from build123d import *

# Parameters (mm, degrees)
F1_DEPTH = 10


with BuildPart() as f1:
    # F0 (on Front) → F1 (new body)
    with BuildSketch(Plane.XZ):
        with BuildLine():
            Line((-30.2, 0), (0, 0))
            Line((0, 0), (0, 1.4))
            Line((0, 1.4), (-15.1, 1.4))
            Line((-15.1, 1.4), (-15.1, 12.9))
            ThreePointArc((-15.1, 12.9), (-15.246447, 13.253553), (-15.6, 13.4))
            ThreePointArc((-15.6, 13.4), (-15.953553, 13.253553), (-16.1, 12.9))
            Line((-16.1, 12.9), (-16.1, 4.4))
            ThreePointArc((-16.1, 4.4), (-16.97868, 2.27868), (-19.1, 1.4))
            Line((-19.1, 1.4), (-28.8, 1.4))
            ThreePointArc((-28.8, 1.4), (-29.789949, 0.989949), (-30.2, 0))
        make_face()
        with BuildLine():
            Line((0, 1.4), (0, 0))
            Line((0, 0), (30.2, 0))
            ThreePointArc((30.2, 0), (29.789949, 0.989949), (28.8, 1.4))
            Line((28.8, 1.4), (19.1, 1.4))
            ThreePointArc((19.1, 1.4), (16.97868, 2.27868), (16.1, 4.4))
            Line((16.1, 4.4), (16.1, 12.9))
            ThreePointArc((16.1, 12.9), (15.953553, 13.253553), (15.6, 13.4))
            ThreePointArc((15.6, 13.4), (15.246447, 13.253553), (15.1, 12.9))
            Line((15.1, 12.9), (15.1, 1.4))
            Line((15.1, 1.4), (0, 1.4))
        make_face()
    extrude(amount=F1_DEPTH)


solid = f1.part
Build history of the part. All positions in model axes, mm. A direction names the side the tool comes from. Round coordinates to 2 decimals unless told otherwise and drop trailing zeros. Write each loop counter-clockwise with the first axis right and the second up, starting at its lowest first coordinate (ties: lowest second). Pieces come first, ordered by that corner, then holes. Notation, with made-up numbers: (81, 0.25) -> (85, 0.25) arc R33 cw to (85, 32.25) -> close; hole circle Ø11 at (55, -27). An arc over 180 degrees is marked (long way). Write item = value, one per line.
(1) Band-saw the part on D-D (x = -2). Give the cut face in (y, z), then the cut area to 3 significant figures.
Answer:
outline = (-10, 0) -> (0, 0) -> (0, 1.4) -> (-10, 1.4) -> close
area = 14.0 mm2
(2) Probe L1, parallel to X at y = -3.5, z = 10.75; L2, parallel to Z at x = -9, y = -5.75; L3, parallel to X at y = -8.25, z = 3.5. List the from-to ranges inside material, lowest first.
Answer:
L1 = -16.1 to -15.1, 15.1 to 16.1
L2 = 0 to 1.4
L3 = -16.24 to -15.1, 15.1 to 16.24
(3) Band-saw the part on B-B (y = -3). Give the cut face in (x, z), then the cut area to 3 significant figures.
Answer:
outline = (-30.2, 0) -> (30.2, 0) arc R1.4 ccw to (28.8, 1.4) -> (19.1, 1.4) arc R3 cw to (16.1, 4.4) -> (16.1, 12.9) arc R0.5 ccw to (15.6, 13.4) arc R0.5 ccw to (15.1, 12.9) -> (15.1, 1.4) -> (-15.1, 1.4) -> (-15.1, 12.9) arc R0.5 ccw to (-15.6, 13.4) arc R0.5 ccw to (-16.1, 12.9) -> (-16.1, 4.4) arc R3 cw to (-19.1, 1.4) -> (-28.8, 1.4) arc R1.4 ccw to start
area = 111 mm2
(4) Band-saw the part on C-C (z = 3.25). Give the cut face in (x, y).
Answer:
outline = (-16.33, -10) -> (-15.1, -10) -> (-15.1, 0) -> (-16.33, 0) -> close; (15.1, -10) -> (16.33, -10) -> (16.33, 0) -> (15.1, 0) -> close
(5) Two-plate mould, pull along X, no slides. Class faces 4 (the face through (-16.1, -5, 9)), 5 (the face through (0, -10, 1)), 6 (the face through (-15.1, -5, 7)): pulls with the +X half, pulls with the -X half, needs draft (parallel to the pull), parting line crosses it, or undercut.
Answer:
face_4 = pulls with the -X half
face_5 = needs draft
face_6 = undercut
(6) Band-saw the part on A-A (z = 6.75). Give the cut face in (x, y).
Answer:
outline = (-16.1, -10) -> (-15.1, -10) -> (-15.1, 0) -> (-16.1, 0) -> close; (15.1, -10) -> (16.1, -10) -> (16.1, 0) -> (15.1, 0) -> close
(7) Tool access for faces 1 (the face through (16.1, -5, 9)), 2 (the face through (15.1, -5, 7)), 3 (the face through (-24, -5, 1.4)): list every direction of +Z, -Z, +X, -X, +Y, -Y with a clear straight run to the whole face (end or side of a thin tool).
Answer:
face_1 = +Z, +X, +Y, -Y
face_2 = +Z, +Y, -Y
face_3 = +Z, -X, +Y, -Y
(8) Flat gauge pins, fed straight in: pin 1 (1.5 mm diameter, centred on y = -6.5, z = 4, fed in from +X); pin 2 (2 mm diameter, centred on y = -8, z = 7, fed in from +X); pin 3 (2 mm diameter, centred on y = -1, z = 2, fed in from +X). Where does each tip first touch, or does it go through?
Answer:
pin_1 = 16.33
pin_2 = 16.1
pin_3 = 29.78
